```python
from build123d import *

# Parameters (mm, degrees)
AUFSATZ_LINEAR_AUSTRAGEN1_DEPTH = 15
SKIZZE8_W                       = 15
SKIZZE8_H                       = 1.8
AUFSATZ_LINEAR_AUSTRAGEN2_DEPTH = 3.6
SKIZZE9_W                       = 1.8
SKIZZE9_H                       = 15
AUFSATZ_LINEAR_AUSTRAGEN3_DEPTH = 1.8
SKIZZE10_W                      = 1.8
SKIZZE10_H                      = 15
AUFSATZ_LINEAR_AUSTRAGEN4_DEPTH = 1.8


# Read off the part's stored shape, not the designer's step: Aufsatz-Linear austragen1
with BuildPart() as part:
    # Aufsatz-Linear austragen1 outline → Aufsatz-Linear austragen1 (new body)
    with BuildSketch(Plane.XY):
        with BuildLine():
            Line((9, 7.5), (9, 5.734326374))
            add(Edge.make_bspline(
                [(9, 5.734326374), (1.374597046, -1.755638023), (8, -9.5)],
                knots=[0.105630562, 0.105630562, 0.105630562, 1, 1, 1], degree=2))
            Line((8, -9.5), (8.759868191, -8.849922825))
            add(Edge.make_bspline(
                [(11, 6.204093636), (10.807716783, 6.040836357), (10.227995606, 5.535038651), (9.02350357, 4.379363864), (7.631707894, 2.723931214), (6.526632736, 0.788286781), (5.948241105, -1.098227765), (5.864634496, -2.960727349), (6.26749431, -4.852517338), (7.040668693, -6.490456848), (7.923606451, -7.821764954), (8.477896684, -8.52033768), (8.759868191, -8.849922825)],
                knots=[0.032316638, 0.032316638, 0.032316638, 0.032316638, 0.0625, 0.125, 0.25, 0.375, 0.5, 0.625, 0.75, 0.875, 0.9375, 1, 1, 1, 1], degree=3))
            Line((11, 6.204093636), (11, 9.5))
            Line((11, 9.5), (-1, 9.5))
            Line((-1, 9.5), (-1, -9.5))
            Line((-1, -9.5), (1, -9.5))
            Line((1, -9.5), (1, 7.5))
            Line((1, 7.5), (9, 7.5))
        make_face()
    extrude(amount=AUFSATZ_LINEAR_AUSTRAGEN1_DEPTH)

    # Skizze8 → Aufsatz-Linear austragen2 (add)
    with BuildSketch(Plane.ZY.offset(1)):
        with Locations((7.5, 8.6)):
            Rectangle(SKIZZE8_W, SKIZZE8_H)
        with Locations((7.5, -8.6)):
            Rectangle(SKIZZE8_W, SKIZZE8_H)
    extrude(amount=AUFSATZ_LINEAR_AUSTRAGEN2_DEPTH)

    # Skizze9 → Aufsatz-Linear austragen3 (add)
    with BuildSketch(Plane(origin=(0, -7.7, 0), x_dir=(1, 0, 0), z_dir=(0, 1, 0))):
        with Locations((-3.7, -7.5)):
            Rectangle(SKIZZE9_W, SKIZZE9_H)
    extrude(amount=AUFSATZ_LINEAR_AUSTRAGEN3_DEPTH)

    # Skizze10 → Aufsatz-Linear austragen4 (add)
    with BuildSketch(Plane.XZ.offset(-7.7)):
        with Locations((-3.7, 7.5)):
            Rectangle(SKIZZE10_W, SKIZZE10_H)
    extrude(amount=AUFSATZ_LINEAR_AUSTRAGEN4_DEPTH)


solid = part.part
```
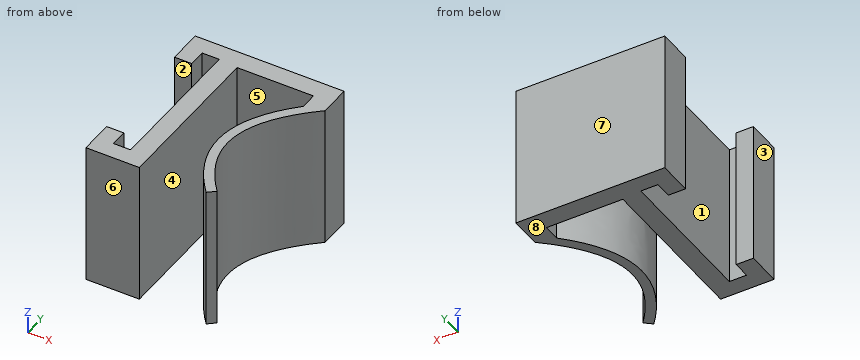
Check sheet for the modelled part. Datum: model origin and axes. Units: mm. Face numbers are marked on the shaded views. A direction names the side the tool comes from. Round coordinates to 2 decimals unless told otherwise and drop trailing zeros. Loops run counter-clockwise (first coordinate to the right, second up) from the corner with the lowest first, then second, coordinate; pieces in that order, holes last. Notation, with made-up numbers: (52.5, -39) -> (85.5, -39) arc R9 ccw to (85.5, -29) -> close; hole circle Ø8 at (-6, -21). An arc over 180 degrees is marked (long way). Answer in a Markdown table with one row per item.
Q1. Sectioned sample at B-B on x = 8.5. Give the number of separate pieces and of enclosed holes in the cut face, then the cut area to 3 significant figures.
Data:
| item | result |
|---|---|
| separate pieces | 3 |
| enclosed holes | 0 |
| area | 60.4 mm^2 |
Q2. Set-up check for the marked faces 1, 2, 3 and 4: record each of +Z, -Z, +X, -X, +Y, -Y from which the full face is reachable in a straight line by a thin tool's end or side.
Data:
| item | result |
|---|---|
| face 1 | +Z, -Z |
| face 2 | +Z, -Z, -X |
| face 3 | +Z, -Z, -X, +Y, -Y |
| face 4 | +Z, -Z, -Y |
Q3. Thickness scan on L1, parallel to X at y = 7, z = 11.25; L2, parallel to Y at x = -1.25, z = 13.5; L3, parallel to X at y = -7, z = 10. Record the ranges inside material, lowest first.
Data:
| item | result |
|---|---|
| L1 | x = -4.6 to -2.8, -1 to 1, 9 to 11 |
| L2 | y = -9.5 to -7.7, 7.7 to 9.5 |
| L3 | x = -4.6 to -2.8, -1 to 1, 6.23 to 7.39 |
Q4. Go/stop test with flat-tipped pins: P1, Ø2, axis at x = 8, z = 6, coming from the -Y side; P2, Ø3, axis at x = -0.5, y = 7, coming from the -Z side; P3, Ø7.5, axis at y = -2, z = 9.5, coming from the -X side; P4, Ø1.5, axis at y = 2.5, z = 1.5, coming from the +X side. Record where each tip stops, or that it passes through.
Data:
| item | result |
|---|---|
| P1 | stops at y = -9.5 |
| P2 | stops at z = 0 |
| P3 | stops at x = -1 |
| P4 | stops at x = 8.11 |
Q5. Release check for a two-part mould opening along Y. For the marked faces 5, 6, 7 and 8 record: released by +Y, released by -Y, zero draft, split by the parting line, or undercut.
Data:
| item | result |
|---|---|
| face 5 | undercut |
| face 6 | released by -Y |
| face 7 | released by +Y |
| face 8 | zero draft |
Q6. Sectioned sample at A-A on x = -3.5. Enter the section's corners in (y, z), then the cut area to 3 significant figures.
Data:
| item | result |
|---|---|
| outline | (-9.5, 0) -> (-5.9, 0) -> (-5.9, 15) -> (-9.5, 15) -> close; (5.9, 0) -> (9.5, 0) -> (9.5, 15) -> (5.9, 15) -> close |
| area | 108 mm^2 |
